Geometry check sheet. Reference: the model listing, model coordinates, mm. Face numbers are marked on the shaded views. A direction names the side the tool comes from. Round coordinates to 2 decimals unless told otherwise and drop trailing zeros. Loops run counter-clockwise (first coordinate to the right, second up) from the corner with the lowest first, then second, coordinate; pieces in that order, holes last. Notation, with made-up numbers: (74, 10.25) - (98, 10.25) arc R10 cw to (98, 16.25) - close; hole circle Ø10 at (3.25, -6). An arc over 180 degrees is marked (long way). Write item = value, one per line.
Solid Edge part; units mm, degrees
sketch "Sketch1" plane through (0, 0, 0) normal (1, 0, 0) x (0, 1, 0)
  line L0 (-59.6342, 10.695) -> (-59.6342, 48.795)
  line L1 (-59.6342, 48.795) -> (-59.6342, 61.495)
  line L2 (-59.6342, 61.495) -> (181.6658, 61.495)
  line L3 (181.6658, 61.495) -> (181.6658, 48.795)
  line L4 (181.6658, 10.695) -> (181.6658, 48.795)
  line L5 (175.3158, 10.695) -> (181.6658, 10.695)
  line L6 (168.6119, 17.3988) -> (175.3158, 10.695)
  line L7 (156.2658, 29.745) -> (168.6119, 17.3988)
  line L8 (137.2158, 10.695) -> (156.2658, 29.745)
  line L9 (-15.1842, 10.695) -> (137.2158, 10.695)
  line L10 (-15.1842, 10.695) -> (-34.2342, 29.745)
  line L11 (-34.2342, 29.745) -> (-53.2842, 10.695)
  line L12 (-53.2842, 10.695) -> (-59.6342, 10.695)
extrude "Protrusion1" add sketch "Sketch1" against normal blind 152.4
sketch "Sketch2" plane through (-76.2, -59.6342, 36.095) normal (0, -1, 0) x (1, 0, 0)
  line L0 (76.2, -76.2) -> (-76.2, -76.2)
  line L1 (-76.2, -76.2) -> (-76.2, 25.4)
  line L2 (-76.2, 25.4) -> (76.2, 25.4)
  line L3 (76.2, 25.4) -> (76.2, -76.2)
extrude "ExtrudedProtrusion_2" add sketch "Sketch2" along normal blind 12.7
sketch "Sketch3" plane through (-76.2, 181.6658, 36.095) normal (0, 1, 0) x (-1, 0, 0)
  line L0 (-76.2, 25.4) -> (76.2, 25.4)
  line L1 (76.2, 25.4) -> (76.2, -25.4)
  line L2 (76.2, -25.4) -> (-76.2, -25.4)
  line L3 (-76.2, -25.4) -> (-76.2, 25.4)
extrude "ExtrudedProtrusion_3" add sketch "Sketch3" along normal blind 12.7
hole "Hole_1" at (-120.65, 61.0158, 61.495) direction (0, 0, -1) diameter 15.875 end up to next counterbore diameter 21.4325 counterbore depth 12.5984
hole "Hole1" at (-31.75, 61.0158, 61.495) direction (0, 0, -1) diameter 15.875 end up to next counterbore diameter 21.4325 counterbore depth 12.5984
sketch "Sketch4" plane through (-76.2, -59.6342, 36.095) normal (0, -1, 0) x (1, 0, 0)
  line L0 (-50.8, 38.1) -> (-38.1, 25.4)
  line L1 (-12.7, 38.1) -> (-50.8, 38.1)
  line L2 (-12.7, 38.1) -> (-12.7, 25.4)
  line L3 (-12.7, 25.4) -> (12.7, 25.4)
  line L4 (12.7, 25.4) -> (12.7, 38.1)
  line L5 (12.7, 38.1) -> (50.8, 38.1)
  line L6 (50.8, 38.1) -> (38.1, 25.4)
extrude "ExtrudedProtrusion_4" add sketch "Sketch4" against normal blind 241.3 material side at (-120.6146, -59.6342, 67.8804)
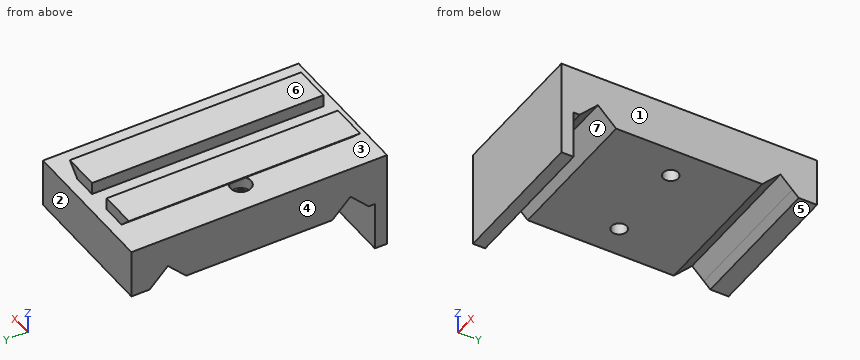
(1) Section check B-B (x = -31.75). Enter the section's corners in (y, z) (3 decimals).
Answers follow:
outline = (-72.334, -40.105) - (-59.634, -40.105) - (-59.634, 10.695) - (-53.284, 10.695) - (-34.234, 29.745) - (-15.184, 10.695) - (53.078, 10.695) - (53.078, 48.897) - (50.3, 48.897) - (50.3, 61.495) - (-72.334, 61.495) - close; (-59.634, 67.845) - (181.666, 67.845) - (181.666, 74.195) - (-59.634, 74.195) - close; (68.953, 10.695) - (137.216, 10.695) - (156.266, 29.745) - (168.612, 17.399) - (175.316, 10.695) - (194.366, 10.695) - (194.366, 61.495) - (71.732, 61.495) - (71.732, 48.897) - (68.953, 48.897) - close
(2) Mould release check, pull along X, two halves, no side actions. Record for the marked faces 1, 2, 3 and 4: pulls with the +X half, pulls with the -X half, needs draft (parallel to the pull), parting line crosses it, or undercut.
Answers follow:
face_1 = pulls with the +X half
face_2 = needs draft
face_3 = undercut
face_4 = pulls with the -X half
(3) Set-up check for the marked faces 5, 6 and 7: record each of +Z, -Z, +X, -X, +Y, -Y from which the full face is reachable in a straight line by a thin tool's end or side.
Answers follow:
face_5 = -Z, +X, -X, +Y
face_6 = +Z, +X, -X, +Y, -Y
face_7 = -Z, +X, -X
(4) Section check C-C (y = 45). Enter the section's corners in (x, z) (3 decimals).
Answers follow:
outline = (-152.4, 10.695) - (0, 10.695) - (0, 61.495) - (-38.1, 61.495) - (-25.4, 74.195) - (-63.5, 74.195) - (-63.5, 61.495) - (-88.9, 61.495) - (-88.9, 74.195) - (-127, 74.195) - (-114.3, 61.495) - (-152.4, 61.495) - close
(5) Gauge pin test, flat ends, axial feed: pin 1 (4 mm diameter, centred on x = -110, z = 69, fed in from +Y); pin 2 (1.9 mm diameter, centred on x = -76.5, y = -55.5, fed in from -Z) (3 decimals); pin 3 (6 mm diameter, centred on x = -16.5, z = -0.5, fed in from +Y). Record the tip position at first contact, or that the pin passes through.
Answers follow:
pin_1 = 181.67
pin_2 = 10.695
pin_3 = -59.63
(6) Scan lines: L1, parallel to Y at x = -31.75, z = 35.5; L2, parallel to Y at x = -31, z = 53; L3, parallel to Y at x = -75, z = 14.5. Record each from-to range of solid material in increasing order. Write a range as [from, to].
Answers follow:
L1 = [-72.33, 53.08], [68.95, 194.37]
L2 = [-72.33, 50.33], [71.71, 194.37]
L3 = [-72.33, -49.48], [-18.99, 141.02], [171.51, 194.37]
(7) Section check A-A (x = -97). Enter the section's corners in (y, z) (3 decimals).
Answers follow:
outline = (-72.334, -40.105) - (-59.634, -40.105) - (-59.634, 10.695) - (-53.284, 10.695) - (-34.234, 29.745) - (-15.184, 10.695) - (137.216, 10.695) - (156.266, 29.745) - (168.612, 17.399) - (175.316, 10.695) - (194.366, 10.695) - (194.366, 61.495) - (181.666, 61.495) - (181.666, 74.195) - (-59.634, 74.195) - (-59.634, 61.495) - (-72.334, 61.495) - close
(8) Section check D-D (z = -5). Enter the section's corners in (x, y).
Answers follow:
outline = (-152.4, -72.33) - (0, -72.33) - (0, -59.63) - (-152.4, -59.63) - close
